from build123d import *

# Parameters (mm, degrees)
SKETCH1_W                      = 20.2
SKETCH1_H                      = 60
SKETCH2_R                      = 20
BOSS_EXTRUDE1_DEPTH            = 4
SKETCH3_R                      = 6
BOSS_EXTRUDE2_DEPTH            = 3
SKETCH4_R                      = 2
BOSS_EXTRUDE3_DEPTH            = 9
SKETCH5_R                      = 20
BOSS_EXTRUDE4_DEPTH            = 4
SKETCH6_R                      = 6.325
BOSS_EXTRUDE5_DEPTH            = 1.5
F_3_3_3_3_DIAMETER_HOLE1_D     = 3.3
F_3_3_3_3_DIAMETER_HOLE1_DEPTH = 8.1
F_3_3_3_3_DIAMETER_HOLE1_TIP   = 0.991420021
CHAMFER1_SIZE                  = 0.3


with BuildPart() as part:
    # Sketch1 → Revolve1 (revolve)
    with BuildSketch(Plane(origin=(0, 0, 0), x_dir=(1, 0, 0), z_dir=(0, 1, 0))):
        with Locations((10.1, 34)):
            Rectangle(SKETCH1_W, SKETCH1_H)
    revolve(axis=Axis((0, 0, -64), (0, 0, 1)))

    # Sketch2 → Boss-Extrude1 (add)
    with BuildSketch(Plane.XY.offset(-4)):
        Circle(SKETCH2_R)
    extrude(amount=BOSS_EXTRUDE1_DEPTH)

    # Sketch3 → Boss-Extrude2 (add)
    with BuildSketch(Plane.XY):
        Circle(SKETCH3_R)
    extrude(amount=BOSS_EXTRUDE2_DEPTH)

    # Sketch4 → Boss-Extrude3 (add)
    with BuildSketch(Plane.XY.offset(3)):
        Circle(SKETCH4_R)
    extrude(amount=BOSS_EXTRUDE3_DEPTH)

    # Sketch5 → Boss-Extrude4 (add)
    with BuildSketch(Plane(origin=(0, 0, -64), x_dir=(-1, 0, 0), z_dir=(0, 0, -1))):
        Circle(SKETCH5_R)
    extrude(amount=BOSS_EXTRUDE4_DEPTH)

    # Sketch6 → Boss-Extrude5 (add)
    with BuildSketch(Plane(origin=(0, 0, -68), x_dir=(-1, 0, 0), z_dir=(0, 0, -1))):
        Circle(SKETCH6_R)
    extrude(amount=BOSS_EXTRUDE5_DEPTH)

    # Ø3.3 (3.3) Diameter Hole1
    with Locations(Plane.XY):
        with Locations((-12.5, 0), (12.5, 0)):
            Hole(F_3_3_3_3_DIAMETER_HOLE1_D / 2, depth=F_3_3_3_3_DIAMETER_HOLE1_DEPTH)
            with Locations((0, 0, -(F_3_3_3_3_DIAMETER_HOLE1_DEPTH + F_3_3_3_3_DIAMETER_HOLE1_TIP / 2))):  # 118° drill point
                Cone(0, F_3_3_3_3_DIAMETER_HOLE1_D / 2, F_3_3_3_3_DIAMETER_HOLE1_TIP, mode=Mode.SUBTRACT)

    # Chamfer1
    chamfer1_edges = [part.edges().sort_by_distance(p)[0] for p in [
        (-6, 0, 3),
        (-2, 0, 12),
        (20, 0, -68),
        (6.325, 0, -69.5),
        (-20, 0, 0),
    ]]
    chamfer(chamfer1_edges, length=CHAMFER1_SIZE)


solid = part.part
Geometry check sheet. Reference: the model listing, model coordinates, mm. A direction names the side the tool comes from. Give positions to 0.01 mm unless a question says otherwise; leave off trailing zeros. Loops run counter-clockwise (first coordinate to the right, second up) from the corner with the lowest first, then second, coordinate; pieces in that order, holes last.
(1) Set-up check for faces 5 (the cylindrical face through (10.976, -0.632, -4.107)), 6 (the flat face through (5, 5, -68)), 7 (the flat face through (0, 0, -69.5)): record each of +Z, -Z, +X, -X, +Y, -Y from which the full face is reachable in a straight line by a thin tool's end or side.
From the geometry:
face 5: +Z
face 6: -Z
face 7: -Z, +X, -X, +Y, -Y
(2) Section check B-B on z = -38. Record the cut outline in (x, y), then the cut area to 3 significant figures.
From the geometry:
outline: circle Ø40.4 at (0, 0)
area: 1,280 mm2
(3) Thickness scan on L1, parallel to Z at x = -10, y = -16; L2, parallel to Y at x = 12, z = -3; L3, parallel to Y at x = 12.5, z = -6. Record the ranges inside material, lowest first.
From the geometry:
L1: z = -68 to 0
L2: y = -16 to -1.57, 1.57 to 16
L3: y = -15.87 to -1.65, 1.65 to 15.87
(4) Release check for a two-part mould opening along X. For faces 1 (the cylindrical face through (1.371, -6.175, -68.592)), 2 (the flat face through (0, 0, 12)), 3 (the conical face through (-12.786, 0.013, -8.919)), 4 (the conical face through (12.214, 0.013, -8.919)) record: released by +X, released by -X, zero draft, split by the parting line, or undercut.
From the geometry:
face 1: split by the parting line
face 2: zero draft
face 3: undercut
face 4: undercut
(5) Depth check by flat-ended pin: pin 1 Ø6 at (x, y) = (7.5, 6) entering from -Z; pin 2 Ø6 at (x, z) = (-9, -54.5) entering from +Y; pin 3 Ø2 at (y, z) = (-2.5, -11.5) entering from +X. Enter the tip coordinate at first touch or a pass-through.
From the geometry:
pin 1: stops at z = -68
pin 2: stops at y = 19.29
pin 3: stops at x = 20.14
